Work out the finished part from the listing and answer in its coordinate system (mm). Face numbers are marked on the shaded views. A direction names the side the tool comes from. Coordinates: 2 decimals unless noted, no trailing zeros. Write each loop counter-clockwise with the first axis right and the second up, starting at its lowest first coordinate (ties: lowest second). Pieces come first, ordered by that corner, then holes. Notation, with made-up numbers: (42, 0) - (96, 0) arc R12 ccw to (96, 6) - close; hole circle Ø6 at (70, 27). An arc over 180 degrees is marked (long way). One line per item, written item: value.
```python
from build123d import *

# Parameters (mm, degrees)
BOSS_EXTRUDE1_DEPTH = 15
SKETCH2_R           = 1.75
SKETCH2_R_2         = 2.25
CUT_EXTRUDE1_DEPTH  = 16.25
SKETCH6_R           = 1.75
CUT_EXTRUDE4_DEPTH  = 51.639881715
SKETCH8_R           = 2.5
CUT_EXTRUDE5_DEPTH  = 2


with BuildPart() as part:
    # Sketch1 → Boss-Extrude1 (new body, symmetric)
    with BuildSketch(Plane.XY):
        with BuildLine():
            Line((25.416367975, 5.477977632), (19.360118285, 31.75))
            Line((19.360118285, 31.75), (22.438796391, 31.75))
            Line((22.438796391, 31.75), (25.127779039, 20.085188295))
            ThreePointArc((25.127779039, 20.085188295), (26.621571391, 17.522387939), (29.304484295, 16.256947461))
            Line((29.304484295, 16.256947461), (36.522421475, 15.243052539))
            ThreePointArc((36.522421475, 15.243052539), (38.256969096, 15.060837158), (40, 15))
            Line((40, 15), (70, 15))
            Line((70, 15), (70, 12))
            Line((70, 12), (62, 12))
            Line((62, 12), (62, 6.75))
            Line((62, 6.75), (70, 6.75))
            Line((70, 6.75), (70, 3.75))
            Line((70, 3.75), (32, 3.75))
            ThreePointArc((32, 3.75), (29.878679656, 2.871320344), (29, 0.75))
            Line((29, 0.75), (29, -0.25))
            Line((29, -0.25), (25.998798049, -0.25))
            ThreePointArc((25.998798049, -0.25), (25.866624369, 2.6301604), (25.416367975, 5.477977632))
        make_face()
    extrude(amount=BOSS_EXTRUDE1_DEPTH, both=True)

    # Sketch2 → Cut-Extrude1 (cut, through all)
    with BuildSketch(Plane(origin=(0, 15, 0), x_dir=(1, 0, 0), z_dir=(0, 1, 0))):
        with Locations((66, 7.5)):
            Circle(SKETCH2_R)
        with Locations((43, 0)):
            Circle(SKETCH2_R_2)
        with Locations((66, -7.5)):
            Circle(SKETCH2_R)
        with BuildLine():
            Line((70, 7.5), (70, 15))
            Line((70, 15), (40, 15))
            Line((40, 15), (66.528351549, 11.464952035))
            ThreePointArc((66.528351549, 11.464952035), (69.009435678, 10.135013644), (70, 7.5))
        make_face()
        with BuildLine():
            Line((40, -15), (66.528351549, -11.464952035))
            ThreePointArc((66.528351549, -11.464952035), (69.009435678, -10.135013644), (70, -7.5))
            Line((70, -7.5), (70, -15))
            Line((70, -15), (40, -15))
        make_face()
    extrude(amount=-CUT_EXTRUDE1_DEPTH, mode=Mode.SUBTRACT)

    # Sketch6 → Cut-Extrude4 (cut, through all)
    with BuildSketch(Plane(origin=(70, 0, 0), x_dir=(0, 0, -1), z_dir=(1, 0, 0))):
        with Locations((-10, 25.75)):
            Circle(SKETCH6_R)
        with Locations((10, 25.75)):
            Circle(SKETCH6_R)
        with BuildLine():
            Line((-10, 30.75), (10, 30.75))
            ThreePointArc((10, 30.75), (13.535533906, 29.285533906), (15, 25.75))
            Line((15, 25.75), (15, 31.75))
            Line((15, 31.75), (-15, 31.75))
            Line((-15, 31.75), (-15, 25.75))
            ThreePointArc((-15, 25.75), (-13.535533906, 29.285533906), (-10, 30.75))
        make_face()
    extrude(amount=-CUT_EXTRUDE4_DEPTH, mode=Mode.SUBTRACT)

    # Sketch8 → Cut-Extrude5 (cut)
    with BuildSketch(Plane(origin=(25, 0, 0), x_dir=(0, 0, -1), z_dir=(1, 0, 0))):
        with Locations((-10, 25.75)):
            Circle(SKETCH8_R)
        with Locations((10, 25.75)):
            Circle(SKETCH8_R)
    extrude(amount=-CUT_EXTRUDE5_DEPTH, mode=Mode.SUBTRACT)


solid = part.part
```
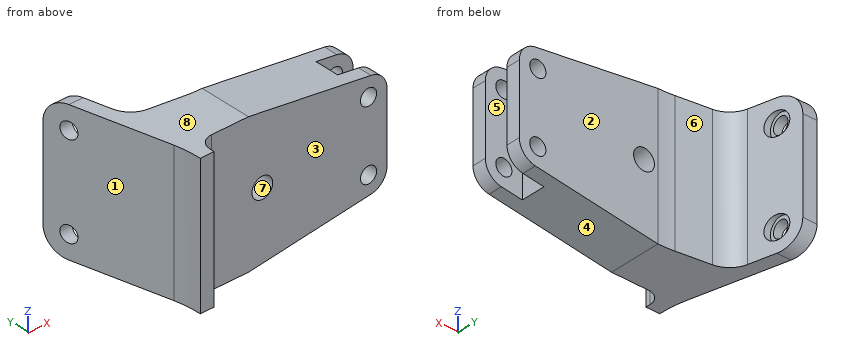
Item 1: Section C-C, the plane x = 43 is taken. Determine the outline of the cut face in (y, z), then the cut area to 3 significant figures.
Evaluation:
outline: (3.75, -14.6) - (15, -14.6) - (15, -2.25) - (3.75, -2.25) - close; (3.75, 2.25) - (15, 2.25) - (15, 14.6) - (3.75, 14.6) - close
area: 278 mm2
Item 2: Section A-A, the plane z = 0 is taken. Determine the outline of the cut face in (x, y), then the cut area to 3 significant figures.
Evaluation:
outline: (19.59, 30.75) - (25.42, 5.48) arc R26 cw to (26, -0.25) - (29, -0.25) - (29, 0.75) arc R3 cw to (32, 3.75) - (40.75, 3.75) - (40.75, 15) - (40, 15) arc R25 cw to (36.52, 15.24) - (29.3, 16.26) arc R5 cw to (25.13, 20.09) - (22.67, 30.75) - close; (45.25, 3.75) - (70, 3.75) - (70, 6.75) - (62, 6.75) - (62, 12) - (70, 12) - (70, 15) - (45.25, 15) - close
area: 494 mm2
Item 3: Determine the mould class of the marked faces 6, 7 and 8 for opening direction X: +X half, -X half, draft (parallel to the pull), parting line (faces both ways), or undercut.
Evaluation:
face 6: +X half
face 7: undercut
face 8: draft
Item 4: Consider probe 1 along Z at (x, y) = (21.2, 25.75); probe 2 along Y at (x, z) = (67, -11.25); probe 3 along Z at (x, y) = (23.65, 25.75). Determine where each line is inside the solid, lowest interval first.
Evaluation:
probe 1: z = -15 to -11.75, -8.25 to 8.25, 11.75 to 15
probe 2: y = 3.75 to 6.75, 12 to 15
probe 3: z = -15 to -12.5, -7.5 to 7.5, 12.5 to 15
Item 5: Section D-D, the plane y = 13.5 is taken. Determine the outline of the cut face in (x, z).
Evaluation:
outline: (23.57, -15) - (40, -15) - (66.53, -11.46) arc R4 ccw to (70, -7.5) - (70, 7.5) arc R4 ccw to (66.53, 11.46) - (40, 15) - (23.57, 15) - close; hole circle Ø4.5 at (43, 0); hole circle Ø3.5 at (66, -7.5); hole circle Ø3.5 at (66, 7.5)
Item 6: Given pin 1 (1.1 mm diameter, centred on y = 0.5, z = 3.5, fed in from +X); pin 2 (5 mm diameter, centred on x = 43, z = 0, fed in from +Y); pin 3 (1.5 mm diameter, centred on y = 9.5, z = -9.5, fed in from +X); pin 4 (3 mm diameter, centred on x = 66, z = 7.5, fed in from -Y), each flat-ended and moving along its own axis, determine where each tip first touches the part or whether it passes through.
Evaluation:
pin 1: stops at x = 29.02
pin 2: stops at y = 15
pin 3: stops at x = 62
pin 4: passes through
Item 7: Which of the six approach directions +Z, -Z, +X, -X, +Y, -Y give full straight-line access (tool end or side, diameter ignored) to the marked faces 1, 2, 3, 4 and 5?
Evaluation:
face 1: +Z, -Z, -X, -Y
face 2: +Z, -Z, +X, +Y
face 3: +Z, -Z, +X, -Y
face 4: -Z, +X, +Y, -Y
face 5: +Z, -Z, +X
Item 8: Section B-B, the plane z = -4.75 is taken. Determine the outline of the cut face in (x, y), then the cut area to 3 significant figures.
Evaluation:
outline: (19.59, 30.75) - (25.42, 5.48) arc R26 cw to (26, -0.25) - (29, -0.25) - (29, 0.75) arc R3 cw to (32, 3.75) - (70, 3.75) - (70, 6.75) - (62, 6.75) - (62, 12) - (70, 12) - (70, 15) - (40, 15) arc R25 cw to (36.52, 15.24) - (29.3, 16.26) arc R5 cw to (25.13, 20.09) - (22.67, 30.75) - close
area: 545 mm2
